Read the model definition and answer for the solid it produces. Units are mm, in the model's axes. A direction names the side the tool comes from. Coordinates: 2 decimals unless noted, no trailing zeros. Write each loop counter-clockwise with the first axis right and the second up, starting at its lowest first coordinate (ties: lowest second). Pieces come first, ordered by that corner, then holes.
1) The part is cut by section B-B (x = -29.5). Determine the outline of the cut face in (y, z), then the cut area to 3 significant figures.
2) Find the intervals of material crossed by line 1 (Y direction, x = -30.5, z = -24); line 2 (X direction, y = -21.5, z = -0.8) (3 decimals); line 3 (Y direction, x = 1.24, z = -1.15) (3 decimals), in increasing order.
3) Determine the mould class of faces 3 (the face through (2, 20, -2.5)), 4 (the face through (-34.1, 31.94, -27.88)), 5 (the face through (-20.515, 22.013, -1.232)) for opening direction X: +X half, -X half, draft (parallel to the pull), parting line (faces both ways), or undercut.
4) Which of the six approach directions +Z, -Z, +X, -X, +Y, -Y give full straight-line access (tool end or side, diameter ignored) to faces 1 (the face through (21.3, 38.7, -2.5)), 2 (the face through (1.045, -22.987, -1.232))?
5) The part is cut by section A-A (z = -30). Determine the outline of the cut face in (x, y), then the cut area to 3 significant figures.
6) Each of these flat-tipped pins is pushed along its axis until it touches: pin 1 Ø6 at (x, y) = (41.53, 11.13) entering from -Z; pin 2 Ø3.5 at (x, y) = (-39, -21.5) entering from -Z; pin 3 Ø5 at (y, z) = (28, -44.5) entering from -X; pin 4 Ø4 at (x, y) = (-4, -12) entering from -Z. Where does it stop, or does it pass through?
from build123d import *

# Parameters (mm, degrees)
SKETCH1_R                    = 47
BOSS_EXTRUDE1_DEPTH          = 2
SKETCH3_R                    = 2.5
CUT_EXTRUDE1_DEPTH           = 67.498120274
BOSS_EXTRUDE2_START          = 55
SKETCH5_R                    = 4
SKETCH5_R_2                  = 2.5
BOSS_EXTRUDE2_DEPTH          = 55
SKETCH2_R                    = 0.825
CUT_EXTRUDE_NANO_RECTO_DEPTH = 88.561407024
SKETCH6_R                    = 1.5
SKETCH6_R_2                  = 0.825
BOSS_EXTRUDE3_DEPTH          = 2.5
SKETCH4_R                    = 0.825
CUT_EXTRUDE_VERSO_DEPTH      = 87.272823067


with BuildPart() as part:
    # Sketch1 → Boss-Extrude1 (new body)
    with BuildSketch(Plane.XY):
        Circle(SKETCH1_R)
    extrude(amount=BOSS_EXTRUDE1_DEPTH)

    # Sketch3 → Cut-Extrude1 (cut, through all)
    with BuildSketch(Plane(origin=(0, 0, 0), x_dir=(-1, 0, 0), z_dir=(0, 0, -1))):
        with Locations((30.405591591, 30.405591591)):
            Circle(SKETCH3_R)
        with Locations((11.129218939, -41.53481053)):
            Circle(SKETCH3_R)
        with Locations((-41.53481053, 11.129218939)):
            Circle(SKETCH3_R)
    extrude(amount=-CUT_EXTRUDE1_DEPTH, mode=Mode.SUBTRACT)

    # Sketch5 → Boss-Extrude2 (add)
    # profile 1 of 3: a face of its own
    with BuildSketch(Plane(origin=(0, 0, 0), x_dir=(-1, 0, 0), z_dir=(0, 0, -1)).offset(BOSS_EXTRUDE2_START)):
        with Locations(Location((30.405591591, 30.405591591, 0), (0, 0, 44.999576406))):
            Circle(SKETCH5_R)
        with Locations((30.405591591, 30.405591591)):
            Circle(SKETCH5_R_2, mode=Mode.SUBTRACT)
    # profile 2 of 3: a face of its own
    with BuildSketch(Plane(origin=(0, 0, 0), x_dir=(-1, 0, 0), z_dir=(0, 0, -1)).offset(BOSS_EXTRUDE2_START)):
        with Locations(Location((11.129218939, -41.53481053, 0), (0, 0, 284.999570993))):
            Circle(SKETCH5_R)
        with Locations((11.129218939, -41.53481053)):
            Circle(SKETCH5_R_2, mode=Mode.SUBTRACT)
    # profile 3 of 3: a face of its own
    with BuildSketch(Plane(origin=(0, 0, 0), x_dir=(-1, 0, 0), z_dir=(0, 0, -1)).offset(BOSS_EXTRUDE2_START)):
        with Locations(Location((-41.53481053, 11.129218939, 0), (0, 0, 164.999581917))):
            Circle(SKETCH5_R)
        with Locations((-41.53481053, 11.129218939)):
            Circle(SKETCH5_R_2, mode=Mode.SUBTRACT)
    extrude(amount=-BOSS_EXTRUDE2_DEPTH)

    # Sketch2 → Cut-Extrude-Nano+Recto (cut, through all)
    with BuildSketch(Plane.XY.offset(2)):
        with Locations((20.32, 38.74)):
            Circle(SKETCH2_R)
        with Locations((20.32, 23.5)):
            Circle(SKETCH2_R)
        with Locations((-20.32, 23.5)):
            Circle(SKETCH2_R)
        with Locations((-20.32, 38.74)):
            Circle(SKETCH2_R)
        with Locations((34.74, 18.98)):
            Circle(SKETCH2_R)
        with Locations((6.26, 18.98)):
            Circle(SKETCH2_R)
        with Locations((-39.24, 18.98)):
            Circle(SKETCH2_R)
        with Locations((1.24, 18.98)):
            Circle(SKETCH2_R)
        with Locations((1.24, -21.5)):
            Circle(SKETCH2_R)
        with Locations((-39.24, -21.5)):
            Circle(SKETCH2_R)
        with BuildLine():
            Line((17.78, 22.875), (-17.78, 22.875))
            ThreePointArc((-17.78, 22.875), (-18.405, 23.5), (-17.78, 24.125))
            Line((-17.78, 24.125), (17.78, 24.125))
            ThreePointArc((17.78, 24.125), (18.405, 23.5), (17.78, 22.875))
        make_face()
        with BuildLine():
            Line((17.78, 39.365), (-17.78, 39.365))
            ThreePointArc((-17.78, 39.365), (-18.405, 38.74), (-17.78, 38.115))
            Line((-17.78, 38.115), (17.78, 38.115))
            ThreePointArc((17.78, 38.115), (18.405, 38.74), (17.78, 39.365))
        make_face()
    extrude(amount=-CUT_EXTRUDE_NANO_RECTO_DEPTH, mode=Mode.SUBTRACT)

    # Sketch6 → Boss-Extrude3 (add)
    # profile 1 of 10: a face of its own
    with BuildSketch(Plane(origin=(0, 0, 0), x_dir=(-1, 0, 0), z_dir=(0, 0, -1))):
        with Locations(Location((-34.74, 18.98, 0), (0, 0, 180))):
            Circle(SKETCH6_R)
        with Locations(Location((-34.74, 18.98, 0), (0, 0, 180))):
            Circle(SKETCH6_R_2, mode=Mode.SUBTRACT)
    # profile 2 of 10: a face of its own
    with BuildSketch(Plane(origin=(0, 0, 0), x_dir=(-1, 0, 0), z_dir=(0, 0, -1))):
        with Locations(Location((-20.32, 23.5, 0), (0, 0, 180))):
            Circle(SKETCH6_R)
        with Locations(Location((-20.32, 23.5, 0), (0, 0, 180))):
            Circle(SKETCH6_R_2, mode=Mode.SUBTRACT)
    # profile 3 of 10: a face of its own
    with BuildSketch(Plane(origin=(0, 0, 0), x_dir=(-1, 0, 0), z_dir=(0, 0, -1))):
        with Locations(Location((-20.32, 38.74, 0), (0, 0, 180))):
            Circle(SKETCH6_R)
        with Locations(Location((-20.32, 38.74, 0), (0, 0, 180))):
            Circle(SKETCH6_R_2, mode=Mode.SUBTRACT)
    # profile 4 of 10: a face of its own
    with BuildSketch(Plane(origin=(0, 0, 0), x_dir=(-1, 0, 0), z_dir=(0, 0, -1))):
        with Locations(Location((20.32, 23.5, 0), (0, 0, 180))):
            Circle(SKETCH6_R)
        with Locations(Location((20.32, 23.5, 0), (0, 0, 180))):
            Circle(SKETCH6_R_2, mode=Mode.SUBTRACT)
    # profile 5 of 10: a face of its own
    with BuildSketch(Plane(origin=(0, 0, 0), x_dir=(-1, 0, 0), z_dir=(0, 0, -1))):
        with Locations(Location((20.32, 38.74, 0), (0, 0, 180))):
            Circle(SKETCH6_R)
        with Locations(Location((20.32, 38.74, 0), (0, 0, 180))):
            Circle(SKETCH6_R_2, mode=Mode.SUBTRACT)
    # profile 6 of 10: a face of its own
    with BuildSketch(Plane(origin=(0, 0, 0), x_dir=(-1, 0, 0), z_dir=(0, 0, -1))):
        with Locations(Location((-6.26, 18.98, 0), (0, 0, 180))):
            Circle(SKETCH6_R)
        with Locations(Location((-6.26, 18.98, 0), (0, 0, 180))):
            Circle(SKETCH6_R_2, mode=Mode.SUBTRACT)
    # profile 7 of 10: a face of its own
    with BuildSketch(Plane(origin=(0, 0, 0), x_dir=(-1, 0, 0), z_dir=(0, 0, -1))):
        with Locations(Location((-1.24, 18.98, 0), (0, 0, 180))):
            Circle(SKETCH6_R)
        with Locations(Location((-1.24, 18.98, 0), (0, 0, 180))):
            Circle(SKETCH6_R_2, mode=Mode.SUBTRACT)
    # profile 8 of 10: a face of its own
    with BuildSketch(Plane(origin=(0, 0, 0), x_dir=(-1, 0, 0), z_dir=(0, 0, -1))):
        with Locations(Location((39.24, 18.98, 0), (0, 0, 180))):
            Circle(SKETCH6_R)
        with Locations(Location((39.24, 18.98, 0), (0, 0, 180))):
            Circle(SKETCH6_R_2, mode=Mode.SUBTRACT)
    # profile 9 of 10: a face of its own
    with BuildSketch(Plane(origin=(0, 0, 0), x_dir=(-1, 0, 0), z_dir=(0, 0, -1))):
        with Locations(Location((39.24, -21.5, 0), (0, 0, 180))):
            Circle(SKETCH6_R)
        with Locations(Location((39.24, -21.5, 0), (0, 0, 180))):
            Circle(SKETCH6_R_2, mode=Mode.SUBTRACT)
    # profile 10 of 10: a face of its own
    with BuildSketch(Plane(origin=(0, 0, 0), x_dir=(-1, 0, 0), z_dir=(0, 0, -1))):
        with Locations(Location((-1.24, -21.5, 0), (0, 0, 180))):
            Circle(SKETCH6_R)
        with Locations(Location((-1.24, -21.5, 0), (0, 0, 180))):
            Circle(SKETCH6_R_2, mode=Mode.SUBTRACT)
    extrude(amount=BOSS_EXTRUDE3_DEPTH)

    # Sketch4 → Cut-Extrude-Verso (cut, through all)
    with BuildSketch(Plane(origin=(0, 0, 0), x_dir=(-1, 0, 0), z_dir=(0, 0, -1))):
        with Locations((-8.26, -36.34)):
            Circle(SKETCH4_R)
        with Locations((2.18, -36.34)):
            Circle(SKETCH4_R)
        with Locations(Location((-26.13, -36.34, 0), (0, 0, 180))):
            Circle(SKETCH4_R)
        with Locations((20.48, -24.54)):
            Circle(SKETCH4_R)
        with BuildLine():
            Line((11.43, -36.34), (11.43, -25.34))
            ThreePointArc((11.43, -25.34), (12.18, -24.59), (12.93, -25.34))
            Line((12.93, -25.34), (12.93, -36.34))
            ThreePointArc((12.93, -36.34), (12.18, -37.09), (11.43, -36.34))
        make_face()
    extrude(amount=-CUT_EXTRUDE_VERSO_DEPTH, mode=Mode.SUBTRACT)


solid = part.part
Reported:
1. outline: (-36.59, 0) - (26.51, 0) - (26.51, -55) - (28.08, -55) - (28.08, 2) - (-36.59, 2) - close; (32.74, -55) - (34.3, -55) - (34.3, 0) - (36.59, 0) - (36.59, 2) - (32.74, 2) - close
1. area: 309 mm2
2. line 1: y = 26.41 to 27.91, 32.9 to 34.4
2. line 2: x = -40.74 to -40.065, -38.415 to -37.74, -0.26 to 0.415, 2.065 to 2.74
2. line 3: y = -23 to -22.325, -20.675 to -20, 17.48 to 18.155, 19.805 to 20.48
3. face 3: draft
3. face 4: parting line
3. face 5: undercut
4. face 1: -Z, +X, -X, +Y, -Y
4. face 2: -Z
5. outline: circle Ø8 at (-30.41, 30.41); circle Ø8 at (-11.13, -41.53); circle Ø8 at (41.53, 11.13); hole circle Ø5 at (-30.41, 30.41); hole circle Ø5 at (-11.13, -41.53); hole circle Ø5 at (41.53, 11.13)
5. area: 91.9 mm2
6. pin 1: stops at z = -55
6. pin 2: stops at z = -2.5
6. pin 3: stops at x = -34.41
6. pin 4: stops at z = 0
